```python
from build123d import *

# Parameters (mm, degrees)
SKETCH1_R           = 6.2865
BOSS_EXTRUDE1_DEPTH = 15.875
SKETCH2_R           = 9.4615
BOSS_EXTRUDE2_DEPTH = 15.875
CUT_EXTRUDE1_DEPTH  = 12.7
FILLET1_R           = 4.7625
SKETCH4_R           = 1.1905
CUT_EXTRUDE2_DEPTH  = 24.398129359


with BuildPart() as part:
    # Sketch1 → Boss-Extrude1 (new body)
    with BuildSketch(Plane(origin=(0, 0, 0), x_dir=(1, 0, 0), z_dir=(0, 1, 0))):
        with Locations(Location((0, 0, 0), (0, 0, 270))):
            Circle(SKETCH1_R)
    extrude(amount=BOSS_EXTRUDE1_DEPTH)

    # Sketch2 → Boss-Extrude2 (add)
    with BuildSketch(Plane(origin=(0, 0, 0), x_dir=(1, 0, 0), z_dir=(0, 1, 0))):
        with Locations(Location((0, 0, 0), (0, 0, 270))):
            Circle(SKETCH2_R)
    extrude(amount=BOSS_EXTRUDE2_DEPTH)

    # Sketch3 → Cut-Extrude1 (cut)
    with BuildSketch(Plane.XZ):
        with BuildLine():
            Line((4.889, -4.248435947), (4.889, 4.248435947))
            ThreePointArc((4.889, 4.248435947), (-6.477, 0), (4.889, -4.248435947))
        make_face()
    extrude(amount=-CUT_EXTRUDE1_DEPTH, mode=Mode.SUBTRACT)

    # Fillet1
    fillet1_edges = [part.edges().sort_by_distance(p)[0] for p in [
        (0, 15.875, -9.4615),
    ]]
    fillet(fillet1_edges, radius=FILLET1_R)

    # Sketch4 → Cut-Extrude2 (cut, through all)
    with BuildSketch(Plane.ZY.offset(-4.889)):
        with Locations((0, 6.35)):
            Circle(SKETCH4_R)
    extrude(amount=-CUT_EXTRUDE2_DEPTH, mode=Mode.SUBTRACT)


solid = part.part
```
Model file for the job. Use its own axes, mm. A direction names the side the tool comes from. Coordinates: 2 decimals unless noted, no trailing zeros. Write each loop counter-clockwise with the first axis right and the second up, starting at its lowest first coordinate (ties: lowest second). Pieces come first, ordered by that corner, then holes. Notation, with made-up numbers: (39.5, 39) - (70.5, 39) arc R25 cw to (70.5, 67) - close; hole circle Ø9 at (-28, 31). An arc over 180 degrees is marked (long way). One line per item, written item: value. Start each with the question number.
1. Slice it at B-B (y = 6.35). Write the cut outline in (x, z), plus the area to 3 significant figures.
2. Slice it at A-A (y = 10). Write the cut outline in (x, z).
3. Tool access for faces 1 (the cylindrical face through (7.14, 7.53, -0.15)), 2 (the cylindrical face through (-6.473, 6.261, 0.22)), 3 (the flat face through (0, 15.875, 0)): list every direction of +Z, -Z, +X, -X, +Y, -Y with a clear straight run to the whole face (end or side of a thin tool).
4. Probe line 1 (X direction, y = 9, z = 0); line 2 (Y direction, x = 3.75, z = -1) (3 decimals); line 3 (X direction, y = 10.25, z = -2.5). List the from-to ranges inside material, lowest first. Write a range as from..to.
5. Mould opens along Z. For faces 4 (the cylindrical face through (2.842, 5.478, 9.025)), 5 (the flat face through (4.889, 8, 0)), 6 (the flat face through (6, 0, 0)) say: released by +Z, released by -Z, zero draft, split by the parting line, or undercut.
6. Flat gauge pins, fed straight in: pin 1 (1.9 mm diameter, centred on y = 6.35, z = 0, fed in from +X); pin 2 (1.5 mm diameter, centred on y = 13, z = -3.5, fed in from -X); pin 3 (8 mm diameter, centred on x = 0, z = 0, fed in from -Y). Where does each tip first touch, or does it go through?
Answers below:
1. outline: (4.89, -4.25) arc R6.48 cw (long way) to (4.89, 4.25) - (4.89, 1.19) - (9.39, 1.19) arc R9.46 ccw (long way) to (9.39, -1.19) - (4.89, -1.19) - close
1. area: 148 mm^2
2. outline: circle Ø18.92 at (0, 0); hole (4.89, -4.25) - (4.89, 4.25) arc R6.48 ccw (long way) to start
3. face 1: +X
3. face 2: -Y
3. face 3: +Z, -Z, +X, -X, +Y
4. line 1: x = -9.46..-6.48, 4.89..9.46
4. line 2: y = 12.7..15.875
4. line 3: x = -9.13..-5.98, 4.89..9.13
5. face 4: split by the parting line
5. face 5: undercut
5. face 6: zero draft
6. pin 1: stops at x = -6.41
6. pin 2: stops at x = -8.78
6. pin 3: stops at y = 12.7
